Verification items for the finished model (mm, model axes). Face numbers are marked on the shaded views. A direction names the side the tool comes from. Give positions to 0.01 mm unless a question says otherwise; leave off trailing zeros. Order: outer loops, then holes, each group sorted by start corner. A loop starts at its lowest first (then second) coordinate and runs counter-clockwise, first axis right, second up. Notation, with made-up numbers: (24.25, 50) -> (55.25, 50) arc R22 ccw to (55.25, 67) -> close; hole circle Ø3 at (-9.75, -18). An arc over 180 degrees is marked (long way). Return JSON: item names as keys, results as strings. Group by question number.
(1) Cross-section at B-B on z = 5. Enter the section's corners in (x, y).
(2) Depth check by flat-ended pin: pin 1 Ø5 at (x, z) = (-5.5, 10) entering from +Y; pin 2 Ø1.5 at (y, z) = (-14, 3.5) entering from -X; pin 3 Ø1 at (x, z) = (-10.5, 6) entering from -Y. Enter the tip coordinate at first touch or a pass-through.
(3) Tool access check on the marked faces 1, 2 and 3. Record the directions out of +Z, -Z, +X, -X, +Y, -Y that give a thin tool (end or side, any length) a straight path to the whole face; none if there is none.
(4) Release check for a two-part mould opening along X. For the marked faces 4, 5 and 6 record: pulls with the +X half, pulls with the -X half, needs draft (parallel to the pull), parting line crosses it, or undercut.
(5) Thickness scan on line 1 along X through (y, z) = (-6.5, 8.5); line 2 along Y through (x, z) = (-3, 11.5); line 3 along X through (y, z) = (10, 11.25). Record the ranges inside material, lowest first.
(6) Cross-section at A-A on x = 0. Enter the section's corners in (y, z) (3 decimals).
from build123d import *

# Parameters (mm, degrees)
ESQUISSE3_R             = 1.6250000000000002
ESQUISSE3_R_2           = 1.6250000000000007
ESQUISSE3_R_3           = 1.625000000000001
ESQUISSE3_R_4           = 6
BOSS_EXTRU_1_DEPTH      = 3.5
ESQUISSE4_R             = 14.499999999999998
ESQUISSE4_R_2           = 7.5
BOSS_EXTRU_2_DEPTH      = 9.524999999999999
CONG_2_R                = 1
CONG_3_R                = 6
ENL_V_MAT_EXTRU_1_DEPTH = 37.971588497459535
ENL_V_MAT_EXTRU_2_DEPTH = 37.971588497459535


with BuildPart() as part:
    # Esquisse3 → Boss.-Extru.1 (new body)
    with BuildSketch(Plane.XY):
        Polygon((0, -31.754264805429408), (-27.499999999999993, 15.877132402714718), (27.500000000000007, 15.877132402714718), align=None)
        with Locations((-17.5, 10.103629710818455)):
            Circle(ESQUISSE3_R, mode=Mode.SUBTRACT)
        with Locations((17.500000000000007, 10.10362971081846)):
            Circle(ESQUISSE3_R_2, mode=Mode.SUBTRACT)
        with Locations((4.24e-15, -20.2072594216369)):
            Circle(ESQUISSE3_R_3, mode=Mode.SUBTRACT)
        Circle(ESQUISSE3_R_4, mode=Mode.SUBTRACT)
    extrude(amount=BOSS_EXTRU_1_DEPTH)

    # Esquisse4 → Boss.-Extru.2 (add)
    with BuildSketch(Plane.XY.offset(3.5)):
        Circle(ESQUISSE4_R)
        Circle(ESQUISSE4_R_2, mode=Mode.SUBTRACT)
    extrude(amount=BOSS_EXTRU_2_DEPTH)

    # Congé2
    cong_2_edges = [part.edges().sort_by_distance(p)[0] for p in [
        (-13.749999999999996, -7.938566201357347, 0),
        (7.11e-15, 15.877132402714718, 0),
        (13.750000000000004, -7.938566201357343, 0),
    ]]
    fillet(cong_2_edges, radius=CONG_2_R)

    # Congé3
    # the kernel refuses this fillet: 6 mm, written as the material it takes off along each edge
    with BuildSketch(Plane(origin=(8.9e-16, -19.754264805429408, 0), x_dir=(0.8660254037844386, -0.5000000000000001, 0), z_dir=(0.5000000000000001, 0.8660254037844386, 0))) as cong_3_piece_1:
        with BuildLine():
            CenterArc((5, -1), 1, 0, 90)
            Line((6, -1), (6, 0))
            Line((6, 0), (5, 0))
        make_face()
    revolve(axis=Axis((8.9e-16, -19.754264805429408, 0), (0, 0, -1)), revolution_arc=120.00000000000001, mode=Mode.SUBTRACT)
    with BuildSketch(Plane(origin=(17.10769515458674, 9.877132402714714, 0), x_dir=(0, 1, 0), z_dir=(-1, 0, 0))) as cong_3_piece_2:
        with BuildLine():
            CenterArc((5, -1), 1, 0, 90)
            Line((6, -1), (6, 0))
            Line((6, 0), (5, 0))
        make_face()
    revolve(axis=Axis((17.10769515458674, 9.877132402714714, 0), (0, 0, -1)), revolution_arc=120.00000000000001, mode=Mode.SUBTRACT)
    with BuildSketch(Plane(origin=(-17.107695154586732, 9.877132402714722, 0), x_dir=(-0.8660254037844387, -0.49999999999999994, 0), z_dir=(0.49999999999999994, -0.8660254037844387, 0))) as cong_3_piece_3:
        with BuildLine():
            CenterArc((5, -1), 1, 0, 90)
            Line((6, -1), (6, 0))
            Line((6, 0), (5, 0))
        make_face()
    revolve(axis=Axis((-17.107695154586732, 9.877132402714722, 0), (0, 0, -1)), revolution_arc=119.99999999999999, mode=Mode.SUBTRACT)
    with BuildSketch(Plane(origin=(-6.7e-16, -31.754264805429408, -2.2e-16), x_dir=(-0.4999999999999999, 0.8660254037844388, 0), z_dir=(0, 0, 1))) as cong_3_piece_4:
        with BuildLine():
            CenterArc((CONG_3_R * 1.73205080757, -CONG_3_R), CONG_3_R, 90.00000000000003, 119.99999999999994)
            Line((CONG_3_R * 0.866025403784, -CONG_3_R * 1.5), (0, 0))
            Line((0, 0), (CONG_3_R * 1.73205080757, 1.1e-16))
        make_face()
    extrude(amount=29.48076211353316, mode=Mode.SUBTRACT)
    with BuildSketch(Plane(origin=(-27.499999999999996, 15.877132402714722, -2.2e-16), x_dir=(0.5, -0.8660254037844386, 0), z_dir=(0, 0, 1))) as cong_3_piece_5:
        with BuildLine():
            CenterArc((CONG_3_R * 1.73205080757, CONG_3_R), CONG_3_R, 150.00000000000003, 119.99999999999997)
            Line((CONG_3_R * 0.866025403784, CONG_3_R * 1.5), (0, 0))
            Line((0, 0), (CONG_3_R * 1.73205080757, 0))
        make_face()
    extrude(amount=29.480762113533153, mode=Mode.SUBTRACT)
    with BuildSketch(Plane(origin=(27.500000000000007, 15.877132402714718, -2.2e-16), x_dir=(-0.5000000000000001, -0.8660254037844385, 0), z_dir=(0, 0, 1))) as cong_3_piece_6:
        with BuildLine():
            CenterArc((CONG_3_R * 1.73205080757, -CONG_3_R), CONG_3_R, 90.00000000000003, 119.99999999999994)
            Line((CONG_3_R * 0.866025403784, -CONG_3_R * 1.5), (0, 0))
            Line((0, 0), (CONG_3_R * 1.73205080757, 1.1e-16))
        make_face()
    extrude(amount=29.480762113533174, mode=Mode.SUBTRACT)

    # Esquisse5 → Enlèv. mat.-Extru.1 (cut, through all)
    with BuildSketch(Plane.XY.offset(13.024999999999999)):
        with BuildLine():
            ThreePointArc((-7.238095238095237, 6.153046182523176), (5.8e-16, 9.499999999999998), (7.238095238095237, 6.153046182523176))
            ThreePointArc((7.238095238095237, 6.153046182523176), (8.647689071844546, 6.038830492462959), (8.761904761904761, 7.448424326212267))
            ThreePointArc((8.761904761904761, 7.448424326212267), (7e-16, 11.5), (-8.761904761904761, 7.448424326212267))
            ThreePointArc((-8.761904761904761, 7.448424326212267), (-8.647689071844544, 6.038830492462961), (-7.238095238095237, 6.153046182523176))
        make_face()
    extrude(amount=-ENL_V_MAT_EXTRU_1_DEPTH, mode=Mode.SUBTRACT)

    # Esquisse6 → Enlèv. mat.-Extru.2 (cut, through all)
    with BuildSketch(Plane.XY.offset(13.024999999999999)):
        with BuildLine():
            ThreePointArc((-2.322580645161291, 5.532234552757338), (-1.3864315887791117, 7.823222318816936), (-3.677419354838709, 8.759371375199114))
            ThreePointArc((-3.677419354838709, 8.759371375199114), (5.8e-16, 9.499999999999998), (3.677419354838709, 8.759371375199114))
            ThreePointArc((3.677419354838709, 8.759371375199114), (1.3864315887791128, 7.823222318816936), (2.322580645161291, 5.532234552757338))
            ThreePointArc((2.322580645161291, 5.532234552757338), (3.7e-16, 6.000000000000003), (-2.322580645161291, 5.532234552757338))
        make_face()
    extrude(amount=-ENL_V_MAT_EXTRU_2_DEPTH, mode=Mode.SUBTRACT)


solid = part.part
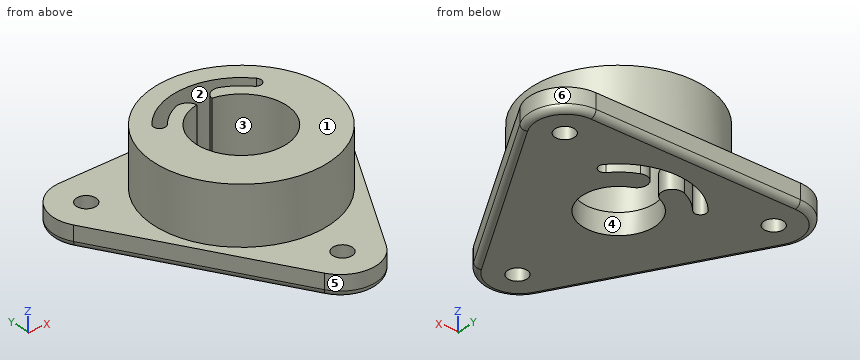
Verdict:
{
 "1": {"outline": "circle Ø29 at (0, 0); hole (-8.76, 7.45) arc R1 ccw to (-7.24, 6.15) arc R9.5 cw to (-3.68, 8.76) arc R1.75 cw to (-1.27, 7.39) arc R7.5 ccw (long way) to (1.27, 7.39) arc R1.75 cw to (3.68, 8.76) arc R9.5 cw to (7.24, 6.15) arc R1 ccw to (8.76, 7.45) arc R11.5 ccw to start"},
 "2": {"pin 1": "y = 14.19", "pin 2": "x = -10.68", "pin 3": "y = -10.5"},
 "3": {"face 1": "+Z, +X, -X, +Y, -Y", "face 2": "+Z, -Z", "face 3": "+Z"},
 "4": {"face 4": "undercut", "face 5": "parting line crosses it", "face 6": "pulls with the +X half"},
 "5": {"line 1": "-12.96 to -3.74, 3.74 to 12.96", "line 2": "-14.19 to -6.87, 6.87 to 8.9, 11.1 to 14.19", "line 3": "-10.5 to -5.68, 5.68 to 10.5"},
 "6": {"outline": "(-25.754, 1) arc R1 ccw to (-24.754, 0) -> (-21.832, 0) -> (-21.832, 3.5) -> (-25.754, 3.5) -> close; (-18.582, 0) -> (-6, 0) -> (-6, 3.5) -> (-7.5, 3.5) -> (-7.5, 13.025) -> (-14.5, 13.025) -> (-14.5, 3.5) -> (-18.582, 3.5) -> close; (11.5, 0) -> (14.877, 0) arc R1 ccw to (15.877, 1) -> (15.877, 3.5) -> (14.5, 3.5) -> (14.5, 13.025) -> (11.5, 13.025) -> close"}
}
